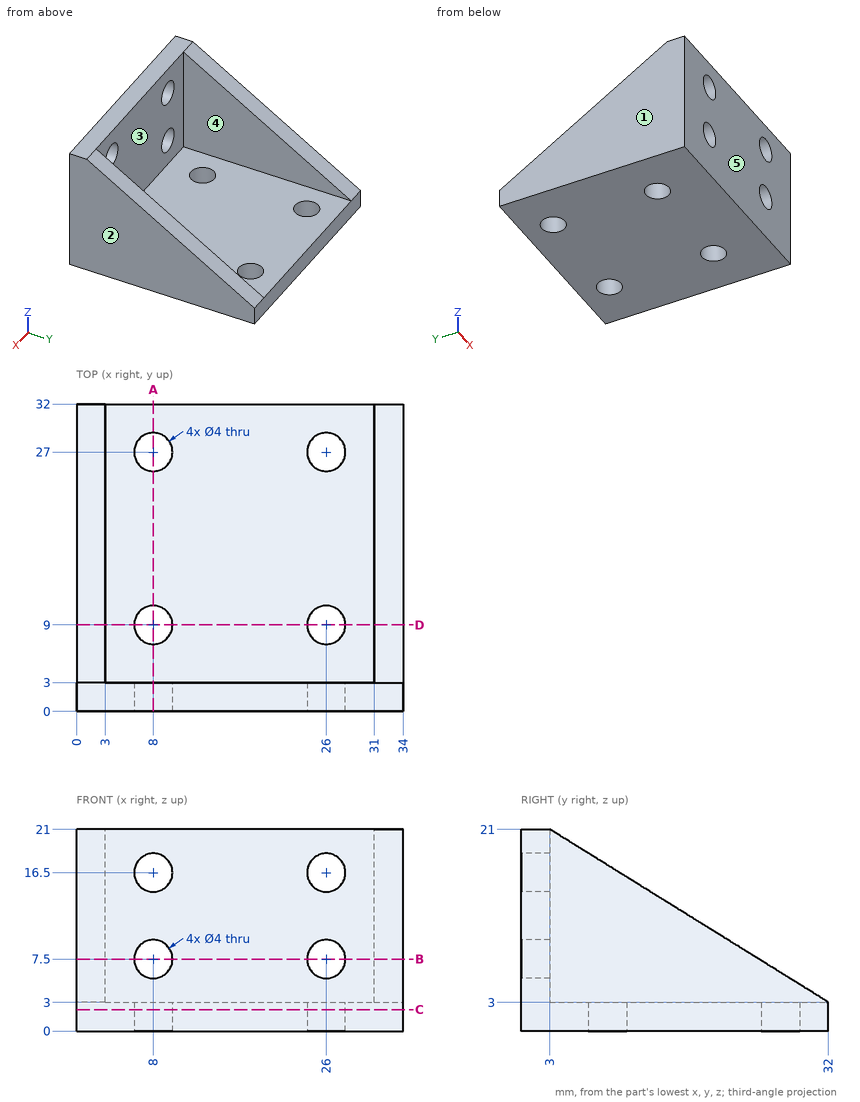
Verification items for this drawing (mm, ordinates from the low corner). A direction names the side the tool comes from. Give positions to 0.01 mm unless a question says otherwise; leave off trailing zeros. Write each loop counter-clockwise with the first axis right and the second up, starting at its lowest first coordinate (ties: lowest second). Pieces come first, ordered by that corner, then holes.
1) Release check for a two-part mould opening along X. For the marked faces 1, 2 and 3 record: pulls with the +X half, pulls with the -X half, needs draft (parallel to the pull), parting line crosses it, or undercut.
2) Section check D-D, the plane y = 9. Record the boundary of the cut face in (x, z), and give its area (3 significant figures).
3) Section check B-B, the plane z = 7.5. Record the boundary of the cut face in (x, y).
4) Section check C-C, the plane z = 2.25. Record the boundary of the cut face in (x, y).
5) Gauge pin test, flat ends, axial feed: pin 1 (10 mm diameter, centred on x = 27.5, z = 12.5, fed in from +Y); pin 2 (6 mm diameter, centred on x = 17.5, z = 13, fed in from +Y); pin 3 (1 mm diameter, centred on x = 15, y = 17.5, fed in from +Z). Record the tip position at first contact, or that the pin passes through.
6) Section check A-A, the plane x = 8. Record the boundary of the cut face in (y, z).
7) Material ranges on L1, parallel to Z at x = 26, y = 1.25; L2, parallel to Y at x = 8, z = 2.35; L3, parallel to Y at x = 5, z = 4.25, recorded low to high.
8) Access from +Z, -Z, +X, -X, +Y, -Y to the whole of each face (thin tool, end or side, straight path). Record for the marked faces 4 and 5.
Computed:
1. face 1: pulls with the -X half
1. face 2: pulls with the +X half
1. face 3: undercut
2. outline: (0, 0) - (6, 0) - (6, 3) - (3, 3) - (3, 17.28) - (0, 17.28) - close; (10, 0) - (24, 0) - (24, 3) - (10, 3) - close; (28, 0) - (34, 0) - (34, 17.28) - (31, 17.28) - (31, 3) - (28, 3) - close
2. area: 164 mm2
3. outline: (0, 0) - (6, 0) - (6, 3) - (3, 3) - (3, 24.75) - (0, 24.75) - close; (10, 0) - (24, 0) - (24, 3) - (10, 3) - close; (28, 0) - (34, 0) - (34, 24.75) - (31, 24.75) - (31, 3) - (28, 3) - close
4. outline: (0, 0) - (34, 0) - (34, 32) - (0, 32) - close; hole circle Ø4 at (8, 9); hole circle Ø4 at (8, 27); hole circle Ø4 at (26, 9); hole circle Ø4 at (26, 27)
5. pin 1: stops at y = 22.45
5. pin 2: stops at y = 3
5. pin 3: stops at z = 3
6. outline: (0, 0) - (7, 0) - (7, 3) - (3, 3) - (3, 5.5) - (0, 5.5) - close; (0, 9.5) - (3, 9.5) - (3, 14.5) - (0, 14.5) - close; (0, 18.5) - (3, 18.5) - (3, 21) - (0, 21) - close; (11, 0) - (25, 0) - (25, 3) - (11, 3) - close; (29, 0) - (32, 0) - (32, 3) - (29, 3) - close
7. L1: z = 0 to 5.5, 9.5 to 14.5, 18.5 to 21
7. L2: y = 0 to 7, 11 to 25, 29 to 32
7. L3: y = 0 to 3
8. face 4: +Z, +Y
8. face 5: +Z, -Z, +X, -X, -Y
